from build123d import *

# Parameters (mm, degrees)
SKETCH2_W           = 8
SKETCH2_H           = 16
BOSS_EXTRUDE1_DEPTH = 6
CUT_EXTRUDE1_DEPTH  = 8
SKETCH4_R           = 1.65
CUT_EXTRUDE2_DEPTH  = 6
FILLET1_R           = 1.5
CHAMFER1_SIZE       = 0.4
CHAMFER2_SIZE       = 0.4


with BuildPart() as part:
    # Sketch2 → Boss-Extrude1 (new body)
    with BuildSketch(Plane.XY):
        Rectangle(SKETCH2_W, SKETCH2_H)
    extrude(amount=BOSS_EXTRUDE1_DEPTH)

    # Sketch3 → Cut-Extrude1 (cut)
    with BuildSketch(Plane.ZY.offset(4)):
        with BuildLine():
            ThreePointArc((0, 1.75), (-1.75, 0), (0, -1.75))
            Line((0, -1.75), (0, 1.75))
        make_face()
        with BuildLine():
            Line((0, 1.75), (0, -1.75))
            ThreePointArc((0, -1.75), (1.237436867, -1.237436867), (1.75, 0))
            ThreePointArc((1.75, 0), (1.237436867, 1.237436867), (0, 1.75))
        make_face()
    extrude(amount=-CUT_EXTRUDE1_DEPTH, mode=Mode.SUBTRACT)

    # Sketch4 → Cut-Extrude2 (cut)
    with BuildSketch(Plane(origin=(0, 0, 0), x_dir=(-1, 0, 0), z_dir=(0, 0, -1))):
        with Locations((0, -4.875)):
            Circle(SKETCH4_R)
        with Locations((0, 4.875)):
            Circle(SKETCH4_R)
    extrude(amount=-CUT_EXTRUDE2_DEPTH, mode=Mode.SUBTRACT)

    # Fillet1
    fillet1_edges = [part.edges().sort_by_distance(p)[0] for p in [
        (4, -8, 3),
        (-4, -8, 3),
        (-4, 8, 3),
        (4, 8, 3),
    ]]
    fillet(fillet1_edges, radius=FILLET1_R)

    # Chamfer1
    chamfer1_edges = [part.edges().sort_by_distance(p)[0] for p in [
        (1.65, -4.875, 6),
        (1.65, 4.875, 6),
        (4, 0, 6),
        (0, -8, 6),
        (0, 8, 6),
        (-4, 0, 6),
        (3.560660172, 7.560660172, 6),
        (-3.560660172, 7.560660172, 6),
        (-3.560660172, -7.560660172, 6),
        (3.560660172, -7.560660172, 6),
    ]]
    chamfer(chamfer1_edges, length=CHAMFER1_SIZE)

    # Chamfer2
    # the kernel refuses this chamfer: 0.4 mm, written as the material it takes off along each edge
    with BuildSketch(Plane(origin=(5.197730184, -1.75, 0), x_dir=(0, 0.1332210476636025, 0.9910863496484109), z_dir=(-1, 0, 0))) as chamfer2_piece_1:
        with BuildLine():
            Line((0.466273667, 0), (-CHAMFER2_SIZE * 0.133221047664, -CHAMFER2_SIZE * 0.991086349648))
            Line((-CHAMFER2_SIZE * 0.133221047664, -CHAMFER2_SIZE * 0.991086349648), (0, 0))
            ThreePointArc((0, 0), (0.23957204, -0.015587056), (0.466273667, 0))
        make_face()
    extrude(amount=10.395460367, mode=Mode.SUBTRACT)
    with BuildSketch(Plane(origin=(-5.197730184, 1.75, 0), x_dir=(0, 1, 0), z_dir=(1, 0, 0))) as chamfer2_piece_2:
        with BuildLine():
            Line((CHAMFER2_SIZE, 0), (-0.062117466, 0.462117466))
            ThreePointArc((-0.062117466, 0.462117466), (-0.01646792, 0.239513102), (0, 0))
            Line((0, 0), (CHAMFER2_SIZE, 0))
        make_face()
    extrude(amount=10.395460367, mode=Mode.SUBTRACT)


solid = part.part
Work out the finished part from the listing and answer in its coordinate system (mm). Round coordinates to 2 decimals unless told otherwise and drop trailing zeros. Write each loop counter-clockwise with the first axis right and the second up, starting at its lowest first coordinate (ties: lowest second). Pieces come first, ordered by that corner, then holes. Notation, with made-up numbers: (44.5, 69) -> (61.5, 69) arc R27 cw to (61.5, 92) -> close; hole circle Ø5 at (41, -25.5). An arc over 180 degrees is marked (long way). Write each question's results on one line, items separated by ' | '.
Item 1: A cutting plane is placed at D-D, the plane y = 1.5. Determine the outline of the cut face in (x, z), plus the area to 3 significant figures.
Result set:
outline: (-4, 0.9) -> (4, 0.9) -> (4, 5.6) -> (3.6, 6) -> (-3.6, 6) -> (-4, 5.6) -> close | area: 40.6 mm^2
Item 2: A flat-ended cylindrical pin translates along its axis: P1, Ø3, axis at x = 1, y = -5, coming from the +Z side. Find the tip coordinate at first contact, or state that the pin passes through.
Result set:
P1: z = 6
Item 3: A cutting plane is placed at A-A, the plane x = 0. Determine the outline of the cut face in (y, z) (3 decimals).
Result set:
outline: (-8, 0) -> (-6.525, 0) -> (-6.525, 5.6) -> (-6.925, 6) -> (-7.6, 6) -> (-8, 5.6) -> close; (-3.225, 0) -> (-2.15, 0) -> (-1.688, 0.462) arc R1.75 cw to (1.688, 0.462) -> (2.15, 0) -> (3.225, 0) -> (3.225, 5.6) -> (2.825, 6) -> (-2.825, 6) -> (-3.225, 5.6) -> close; (6.525, 0) -> (8, 0) -> (8, 5.6) -> (7.6, 6) -> (6.925, 6) -> (6.525, 5.6) -> close
Item 4: A cutting plane is placed at B-B, the plane z = 1. Determine the outline of the cut face in (x, y) (3 decimals).
Result set:
outline: (-4, -6.5) arc R1.5 ccw to (-2.5, -8) -> (2.5, -8) arc R1.5 ccw to (4, -6.5) -> (4, -1.436) -> (-4, -1.436) -> close; (-4, 1.436) -> (4, 1.436) -> (4, 6.5) arc R1.5 ccw to (2.5, 8) -> (-2.5, 8) arc R1.5 ccw to (-4, 6.5) -> close; hole circle Ø3.3 at (0, -4.875); hole circle Ø3.3 at (0, 4.875)
Item 5: The mould has two halves that part along Y. Classify faces 1 (the face through (-3.57, 7.55, 2.84)), 2 (the face through (-3.57, -7.55, 2.84)), 3 (the face through (0.358, 3.264, 2.761)): +Y half, -Y half, draft (parallel to the pull), parting line (faces both ways), or undercut.
Result set:
face 1: +Y half | face 2: -Y half | face 3: undercut
Item 6: A cutting plane is placed at C-C, the plane z = 5. Determine the outline of the cut face in (x, y) (3 decimals).
Result set:
outline: (-4, -6.5) arc R1.5 ccw to (-2.5, -8) -> (2.5, -8) arc R1.5 ccw to (4, -6.5) -> (4, 6.5) arc R1.5 ccw to (2.5, 8) -> (-2.5, 8) arc R1.5 ccw to (-4, 6.5) -> close; hole circle Ø3.3 at (0, -4.875); hole circle Ø3.3 at (0, 4.875)
Item 7: Find the intervals of material crossed by line 1 along Y through (x, z) = (0, 3.7) (3 decimals); line 2 along Y through (x, z) = (-0.5, 4.5); line 3 along Y through (x, z) = (0, 1.4) (3 decimals), in increasing order. Write a range as [from, to].
Result set:
line 1: [-8, -6.525], [-3.225, 3.225], [6.525, 8] | line 2: [-8, -6.45], [-3.3, 3.3], [6.45, 8] | line 3: [-8, -6.525], [-3.225, -1.05], [1.05, 3.225], [6.525, 8]
